Study the drawing (mm; zero at the part's minimum x, y, z) and answer. Coordinates: 2 decimals unless noted, no trailing zeros. Loops run counter-clockwise (first coordinate to the right, second up) from the corner with the lowest first, then second, coordinate; pieces in that order, holes last. Notation, with made-up numbers: (64, 74.25) - (92, 74.25) arc R23 cw to (92, 104.25) - close; hole circle Ø3 at (-15.5, 10). An arc over 180 degrees is marked (long way). One line per item, written item: value. Start each with the question number.
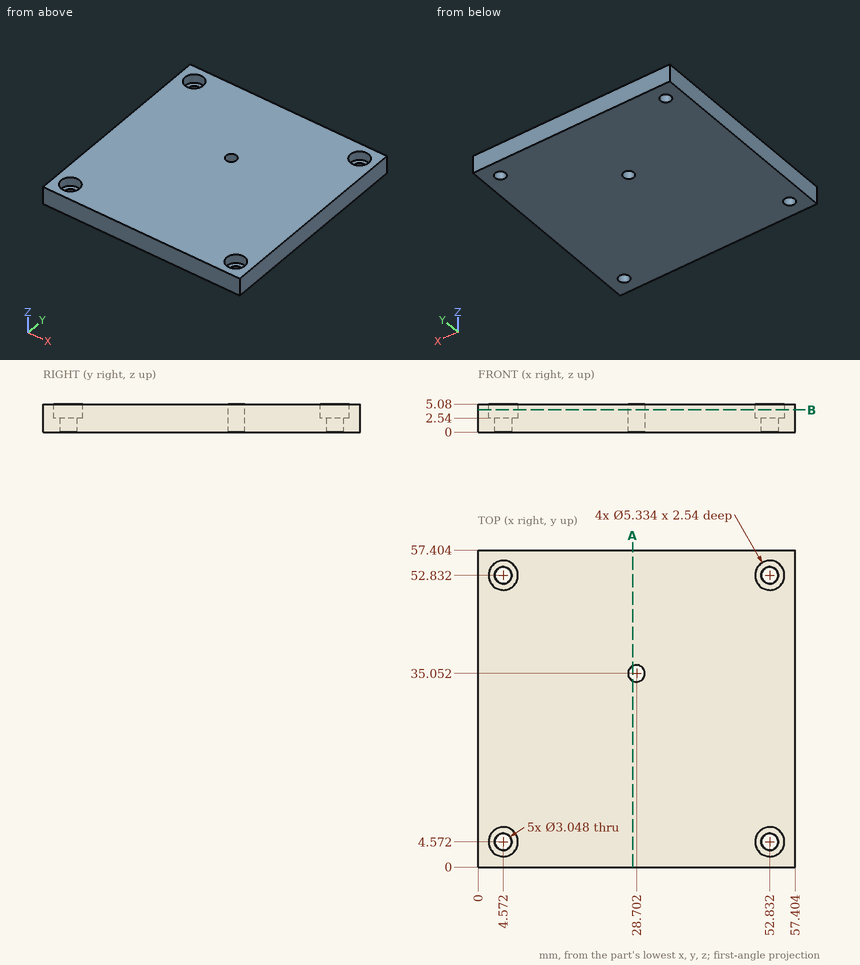
1) Straight lines are drawn through the part: L1, parallel to X at y = 53, z = 1.2; L2, parallel to Y at x = 3, z = 4.3. For each, find the intervals that lie inside material, in ascending order.
2) Section A-A, the plane x = 28 is taken. Determine the outline of the cut face in (y, z).
3) A flat-ended cylindrical pin translates along its axis: P1, Ø2.5, axis at x = 52.5, y = 52.5, coming from the +Z side. Find the tip coordinate at first contact, or state that the pin passes through.
4) Section B-B, the plane z = 4 is taken. Determine the outline of the cut face in (x, y), and give its area (3 significant figures).
Answer below:
1. L1: 0 to 3.06, 6.09 to 51.32, 54.35 to 57.4
1. L2: 0 to 2.42, 6.73 to 50.68, 54.99 to 57.4
2. outline: (0, 0) - (33.7, 0) - (33.7, 5.08) - (0, 5.08) - close; (36.4, 0) - (57.4, 0) - (57.4, 5.08) - (36.4, 5.08) - close
3. P1: z = 2.54
4. outline: (0, 0) - (57.4, 0) - (57.4, 57.4) - (0, 57.4) - close; hole circle Ø5.33 at (4.57, 4.57); hole circle Ø5.33 at (4.57, 52.83); hole circle Ø3.05 at (28.7, 35.05); hole circle Ø5.33 at (52.83, 4.57); hole circle Ø5.33 at (52.83, 52.83)
4. area: 3,200 mm2
